Could you check a few things on this model? Use its own coordinates, in mm. Face numbers are marked on the shaded views. A direction names the side the tool comes from. Give positions to 0.01 mm unless a question says otherwise; leave off trailing zeros. Loops run counter-clockwise (first coordinate to the right, second up) from the corner with the lowest first, then second, coordinate; pieces in that order, holes last. Notation, with made-up numbers: (28, 2.25) - (68, 2.25) arc R21 ccw to (68, 16.25) - close; hole circle Ø9 at (-11, 13.5). An arc over 180 degrees is marked (long way). Write each question's results on one line, items separated by ' | '. Start each with the question number.
1) I'm going to push flat-ended pins straight in: pin 1 (2.5 mm diameter, centred on x = 1.5, y = -0.5, fed in from +Z); pin 2 (4 mm diameter, centred on y = 4, z = 5, fed in from -X); pin 3 (8 mm diameter, centred on y = -5, z = 18.5, fed in from +X). Where does each tip first touch, or does it pass through?
2) If I drill on probe 1 along Y at (x, z) = (0, 15.5); probe 2 along Y at (x, z) = (0, 3.5); probe 3 along X at (y, z) = (-2.25, 10.75), over which ranges is the centre line in solid material (lowest first)? Write a range as [from, to].
3) I want a section at A-A, the plane y = 0. Write out the boundary of the cut face in (x, z), and give its area (3 significant figures).
4) On a 3-axis mill with a long thin cutter (end or side, diameter ignored), from which of +Z, -Z, +X, -X, +Y, -Y can I reach the whole of each face in a straight line? I mean the marked faces 4 and 5. Say none if no direction works.
5) If we mould it in two halves opening along Y, with no side actions, what happens to the marked faces 1, 2 and 3? For each: +Y half, -Y half, draft (parallel to the pull), parting line (faces both ways), or undercut.
6) I want a section at C-C, the plane z = 9.75. Write out the boundary of the cut face in (x, y), and give its area (3 significant figures).
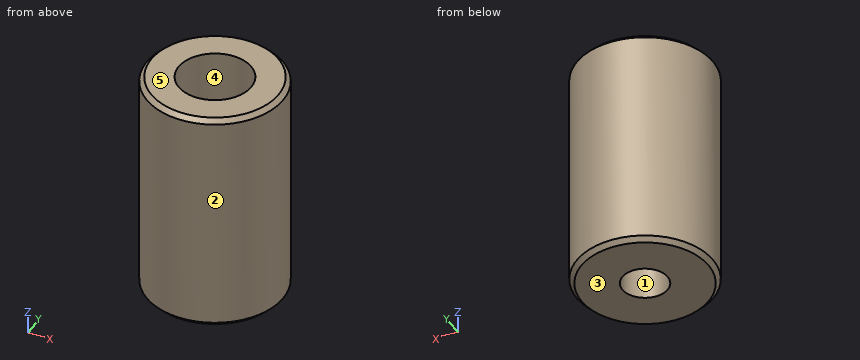
from build123d import *

# Parameters (mm, degrees)
F0_R     = 7.5
F0_R_2   = 4
F1_DEPTH = 25
F0_R_3   = 2.5
F2_DEPTH = 12.5
F3_DEPTH = 12.5
F4_SIZE  = 0.5


with BuildPart() as f1:
    # F0 (on Top) → F1 (new body)
    with BuildSketch(Plane.XY):
        Circle(F0_R)
        Circle(F0_R_2, mode=Mode.SUBTRACT)
    extrude(amount=F1_DEPTH)

    # F0 (on Top) → F2 (join)
    with BuildSketch(Plane.XY):
        Circle(F0_R_3)
        Circle(F0_R_2)
        Circle(F0_R_3, mode=Mode.SUBTRACT)
    extrude(amount=F2_DEPTH)

    # F0 (on Top) → F3 (cut)
    with BuildSketch(Plane.XY):
        Circle(F0_R_3)
    extrude(amount=F3_DEPTH, mode=Mode.SUBTRACT)

    # F4
    f4_edges = [f1.edges().sort_by_distance(p)[0] for p in [
        (-7.5, 0, 25),
        (-7.5, 0, 0),
    ]]
    chamfer(f4_edges, length=F4_SIZE)


solid = f1.part
Answers:
1) pin 1: stops at z = 12.5 | pin 2: stops at x = -7.23 | pin 3: stops at x = 7.43
2) probe 1: y = [-7.5, -4], [4, 7.5] | probe 2: y = [-7.5, -2.5], [2.5, 7.5] | probe 3: x = [-7.15, -1.09], [1.09, 7.15]
3) outline: (-7.5, 0.5) - (-7, 0) - (-2.5, 0) - (-2.5, 12.5) - (-4, 12.5) - (-4, 25) - (-7, 25) - (-7.5, 24.5) - close; (2.5, 0) - (7, 0) - (7.5, 0.5) - (7.5, 24.5) - (7, 25) - (4, 25) - (4, 12.5) - (2.5, 12.5) - close | area: 212 mm2
4) face 4: +Z | face 5: +Z, +X, -X, +Y, -Y
5) face 1: undercut | face 2: parting line | face 3: draft
6) outline: circle Ø15 at (0, 0); hole circle Ø5 at (0, 0) | area: 157 mm2
